Work out the finished part from the listing and answer in its coordinate system (mm). Face numbers are marked on the shaded views. A direction names the side the tool comes from. Give positions to 0.01 mm unless a question says otherwise; leave off trailing zeros. Write each loop counter-clockwise with the first axis right and the second up, starting at its lowest first coordinate (ties: lowest second). Pieces come first, ordered by that corner, then holes. Notation, with made-up numbers: (0.25, -2) - (40.25, -2) arc R26 cw to (40.25, 21) - close; hole circle Ø5 at (-33.5, -10). An arc over 180 degrees is marked (long way). Write item = value, one per line.
from build123d import *

# Parameters (mm, degrees)
SKETCH1_R           = 11.5
BOSS_EXTRUDE1_DEPTH = 10
SKETCH2_R           = 8.5
CUT_EXTRUDE2_DEPTH  = 10
SKETCH4_R           = 4
BOSS_EXTRUDE2_DEPTH = 10
BOSS_EXTRUDE3_START = 10
BOSS_EXTRUDE3_DEPTH = 10
CIRPATTERN1_COUNT   = 5
CUT_EXTRUDE4_DEPTH  = 10
SKETCH8_R           = 1.75
BOSS_EXTRUDE4_DEPTH = 2
CUT_EXTRUDE5_DEPTH  = 2
FILLET1_R           = 2.25


with BuildPart() as part:
    # Sketch1 → Boss-Extrude1 (new body)
    with BuildSketch(Plane.XY):
        Circle(SKETCH1_R)
    extrude(amount=BOSS_EXTRUDE1_DEPTH)

    # Sketch2 → Cut-Extrude2 (cut)
    with BuildSketch(Plane.XY.offset(10)):
        Circle(SKETCH2_R)
    extrude(amount=-CUT_EXTRUDE2_DEPTH, mode=Mode.SUBTRACT)



with BuildPart() as body_2:
    # Sketch4 → Boss-Extrude2 (new body)
    with BuildSketch(Plane.XY):
        Circle(SKETCH4_R)
    extrude(amount=BOSS_EXTRUDE2_DEPTH)


with BuildPart() as part_1:
    add(part.part)

    add(body_2.part)  # Boss-Extrude3 merges body 2
    # Sketch6 → Boss-Extrude3 (add)
    with BuildSketch(Plane.XY.offset(BOSS_EXTRUDE3_START)):
        with BuildLine():
            Line((-1.114437127, 3.841618134), (-2.368178894, 8.163438536))
            ThreePointArc((-2.368178894, 8.163438536), (-0.122551325, 8.499116494), (2.131821106, 8.228325393))
            Line((2.131821106, 8.228325393), (0.940332104, 3.887901173))
            ThreePointArc((0.940332104, 3.887901173), (-0.090075911, 3.998985663), (-1.114437127, 3.841618134))
        make_face()
    boss_extrude3 = extrude(amount=-BOSS_EXTRUDE3_DEPTH)

    # CirPattern1: Boss-Extrude3 ×5 about axis
    cirpattern1_axis = Axis((0, 0, 0), (0, 0, 1))
    for i in range(1, CIRPATTERN1_COUNT):
        add(boss_extrude3.rotate(cirpattern1_axis, i * 360 / CIRPATTERN1_COUNT))

    # Sketch7 → Cut-Extrude4 (cut)
    with BuildSketch(Plane.XY.offset(10)):
        with BuildLine():
            Line((-1.118033989, 1), (1.118033989, 1))
            ThreePointArc((1.118033989, 1), (0, -1.5), (-1.118033989, 1))
        make_face()
    extrude(amount=-CUT_EXTRUDE4_DEPTH, mode=Mode.SUBTRACT)

    # Sketch8 → Boss-Extrude4 (add)
    with BuildSketch(Plane.XY.offset(10)):
        Circle(SKETCH8_R)
    extrude(amount=BOSS_EXTRUDE4_DEPTH)

    # Sketch9 → Cut-Extrude5 (cut)
    with BuildSketch(Plane.XY.offset(12)):
        with BuildLine():
            Line((-1.118033989, 1), (1.118033989, 1))
            ThreePointArc((1.118033989, 1), (0, -1.5), (-1.118033989, 1))
        make_face()
    extrude(amount=-CUT_EXTRUDE5_DEPTH, mode=Mode.SUBTRACT)

    # Fillet1
    # the kernel refuses this fillet: 2.25 mm, written as the material it adds along each edge
    with BuildSketch(Plane(origin=(0, 0, 10), x_dir=(1, 0, 0), z_dir=(0, -1, 0))) as fillet1_piece_1:
        with BuildLine():
            CenterArc((3.986067977, 2.25), FILLET1_R, 186.379370208, 83.620629792)
            Line((1.75, 2), (1.70527864, 1.995))
            ThreePointArc((1.70527864, 1.995), (1.705, 1), (1.705, 0))
            Line((1.705, 0), (1.75, -0.045))
            Line((1.75, -0.045), (3.986067977, -0.045))
            Line((3.986067977, -0.045), (3.986067977, 0))
        make_face()
    revolve(axis=Axis((0, 0, 10), (0, 0, 1)))


solid = part_1.part
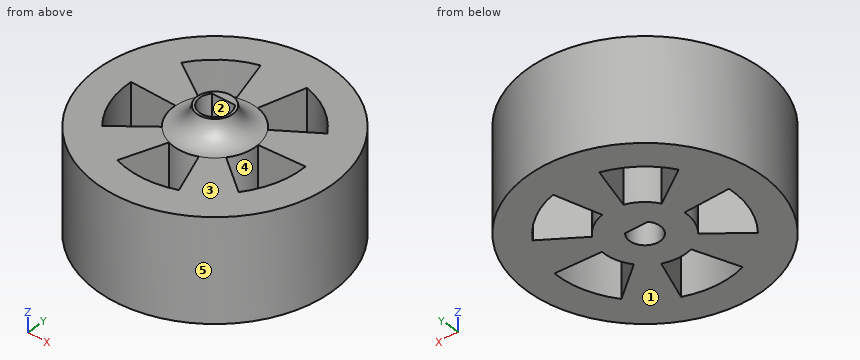
1. Find section B-B, the plane y = 7.75. Give the vertices of the cut face in (x, z), then the cut area to 3 significant figures.
Solution:
outline = (-8.5, 0) - (-3.49, 0) - (-3.49, 10) - (-8.5, 10) - close; (-2.25, 0) - (2, 0) - (2, 10) - (-2.25, 10) - close; (3.49, 0) - (8.5, 0) - (8.5, 10) - (3.49, 10) - close
area = 143 mm^2
2. Straight lines are drawn through the part: line 1 (X direction, y = -1.25, z = 9.25); line 2 (Y direction, x = -5, z = 4.75); line 3 (Z direction, x = 4.5, y = 0.75). For each, find the intervals that lie inside material, in ascending order.
Solution:
line_1 = -11.43 to -8.41, -3.8 to -0.83, 0.83 to 3.8, 8.41 to 11.43
line_2 = -10.36 to -4.16, 0.16 to 3.14, 6.87 to 10.36
line_3 = 0 to 10
3. A tool of negligible diameter and unlimited length cuts with its end or side. For the marked faces 1 and 2, from which of +Z, -Z, +X, -X, +Y, -Y can it reach the whole face along a straight path? Write none if from no direction.
Solution:
face_1 = -Z, +X, -X, +Y, -Y
face_2 = +Z, -Z
4. Given pin 1 (7 mm diameter, centred on x = 5.5, y = -1, fed in from +Z); pin 2 (6 mm diameter, centred on x = 8, z = 10.5, fed in from +Y); pin 3 (2 mm diameter, centred on x = 5, z = 10, fed in from +Y), each flat-ended and moving along its own axis, determine where each tip first touches the part or whether it passes through.
Solution:
pin_1 = 11.04
pin_2 = 10.34
pin_3 = 10.78
5. For a pull along Y with two mould halves and no side action, classify the marked faces 3, 4 and 5 as pulls with the +Y half, pulls with the -Y half, needs draft (parallel to the pull), parting line crosses it, or undercut.
Solution:
face_3 = needs draft
face_4 = undercut
face_5 = parting line crosses it
6. Find section C-C, the plane z = 4. Give the vertices of the cut face in (x, y), then the cut area to 3 significant figures.
Solution:
outline = circle Ø23 at (0, 0); hole (-8.5, 0.27) arc R8.5 ccw to (-6.56, -5.4) - (-3.05, -2.59) arc R4 cw to (-4, 0.13) - close; hole (-7.17, 4.57) - (-3.41, 2.1) arc R4 cw to (-1.11, 3.84) - (-2.37, 8.16) arc R8.5 ccw to start; hole (-2.88, -8) arc R8.5 ccw to (3.11, -7.91) - (1.52, -3.7) arc R4 cw to (-1.36, -3.76) - close; hole (-1.12, 1) arc R1.5 ccw (long way) to (1.12, 1) - close; hole (0.94, 3.89) arc R4 cw to (3.31, 2.25) - (7.03, 4.77) arc R8.5 ccw to (2.13, 8.23) - close; hole (3.16, -2.45) - (6.71, -5.21) arc R8.5 ccw to (8.48, 0.52) - (3.99, 0.31) arc R4 cw to start
area = 307 mm^2
7. Find section D-D, the plane x = 4.5. Give the vertices of the cut face in (y, z), then the cut area to 3 significant figures.
Solution:
outline = (-10.58, 0) - (-3.49, 0) - (-3.49, 10) - (-10.58, 10) - close; (0.33, 0) - (3.06, 0) - (3.06, 10) - (0.33, 10) - close; (7.21, 0) - (10.58, 0) - (10.58, 10) - (7.21, 10) - close
area = 132 mm^2
8. Find section A-A, the plane x = 0. Give the number of separate pieces and of enclosed holes in the cut face, then the cut area to 3 significant figures.
Solution:
separate_pieces = 3
enclosed_holes = 0
area = 164 mm^2
